The figure shows three views and two pictorial views of one solid part (mm, origin at its lowest corner). Answer the questions. A direction names the side the tool comes from. Coordinates: 2 decimals unless noted, no trailing zeros. Write each loop counter-clockwise with the first axis right and the second up, starting at its lowest first coordinate (ties: lowest second). Pieces come first, ordered by that corner, then holes.
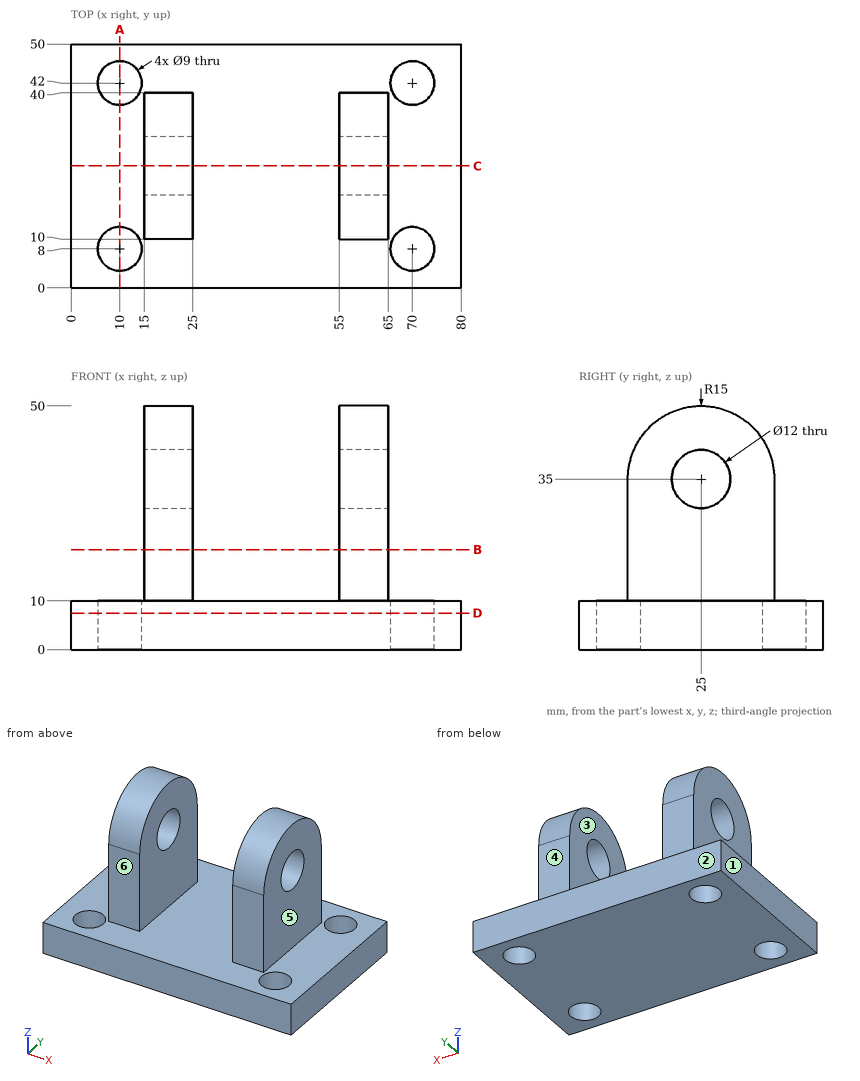
Item 1: The part is cut by section C-C (y = 25). Give the vertices of the cut face in (x, z).
Item 2: The part is cut by section A-A (x = 10). Give the vertices of the cut face in (y, z), and give its area (3 significant figures).
Item 3: The part is cut by section D-D (z = 7.5). Give the vertices of the cut face in (x, y), and give its area (3 significant figures).
Item 4: Given pin 1 (11 mm diameter, centred on x = 59, z = 17.5, fed in from -Y); pin 2 (7 mm diameter, centred on x = 10, y = 8, fed in from +Z); pin 3 (15 mm diameter, centred on y = 32, z = 30.5, fed in from +X); pin 4 (5 mm diameter, centred on x = 56.5, z = 33, fed in from +Y), each flat-ended and moving along its own axis, determine where each tip first touches the part or whether it passes through.
Item 5: Determine the mould class of the marked faces 1, 2 and 3 for opening direction X: +X half, -X half, draft (parallel to the pull), parting line (faces both ways), or undercut.
Item 6: The part is cut by section B-B (z = 20.5). Give the vertices of the cut face in (x, y), and give its area (3 significant figures).
Item 7: Find the intervals of material crossed by probe 1 along X at (y, z) = (8, 4.25); probe 2 along Y at (x, z) = (70, 3.5); probe 3 along Z at (x, y) = (21, 25), in increasing order.
Item 8: For the marked faces 4, 5 and 6, determine the directions among +Z, -Z, +X, -X, +Y, -Y from which every point of the face is accessible in a straight line to the end or side of a thin tool.
Answer:
1. outline: (0, 0) - (80, 0) - (80, 10) - (65, 10) - (65, 29) - (55, 29) - (55, 10) - (25, 10) - (25, 29) - (15, 29) - (15, 10) - (0, 10) - close; (15, 41) - (25, 41) - (25, 50) - (15, 50) - close; (55, 41) - (65, 41) - (65, 50) - (55, 50) - close
2. outline: (0, 0) - (3.5, 0) - (3.5, 10) - (0, 10) - close; (12.5, 0) - (37.5, 0) - (37.5, 10) - (12.5, 10) - close; (46.5, 0) - (50, 0) - (50, 10) - (46.5, 10) - close
2. area: 320 mm2
3. outline: (0, 0) - (80, 0) - (80, 50) - (0, 50) - close; hole circle Ø9 at (10, 8); hole circle Ø9 at (10, 42); hole circle Ø9 at (70, 8); hole circle Ø9 at (70, 42)
3. area: 3,750 mm2
4. pin 1: stops at y = 10
4. pin 2: passes through
4. pin 3: stops at x = 65
4. pin 4: stops at y = 40
5. face 1: -X half
5. face 2: draft
5. face 3: undercut
6. outline: (15, 10) - (25, 10) - (25, 40) - (15, 40) - close; (55, 10) - (65, 10) - (65, 40) - (55, 40) - close
6. area: 600 mm2
7. probe 1: x = 0 to 5.5, 14.5 to 65.5, 74.5 to 80
7. probe 2: y = 0 to 3.5, 12.5 to 37.5, 46.5 to 50
7. probe 3: z = 0 to 29, 41 to 50
8. face 4: +Z, +X, -X, +Y
8. face 5: +Z, +X, +Y, -Y
8. face 6: +Z, +X, -X, -Y
